```python
from build123d import *

# Parameters (mm, degrees)
SKETCH1_W           = 825.5
SKETCH1_H           = 825.5
SKETCH1_W_2         = 647.7
SKETCH1_H_2         = 647.7
BOSS_EXTRUDE1_DEPTH = 127
FILLET1_R           = 25.4
FILLET2_R           = 12.7
SKETCH2_W           = 34.200403136
SKETCH2_H           = 9.659395297
CUT_EXTRUDE1_DEPTH  = 5.08


with BuildPart() as part:
    # Sketch1 → Boss-Extrude1 (new body)
    with BuildSketch(Plane(origin=(0, 0, 0), x_dir=(1, 0, 0), z_dir=(0, 1, 0))):
        Rectangle(SKETCH1_W, SKETCH1_H)
        Rectangle(SKETCH1_W_2, SKETCH1_H_2, mode=Mode.SUBTRACT)
    extrude(amount=BOSS_EXTRUDE1_DEPTH)

    # Fillet1
    fillet1_edges = [part.edges().sort_by_distance(p)[0] for p in [
        (412.75, 63.5, 412.75),
        (-412.75, 63.5, 412.75),
        (-412.75, 63.5, -412.75),
        (412.75, 63.5, -412.75),
    ]]
    fillet(fillet1_edges, radius=FILLET1_R)

    # Fillet2
    fillet2_edges = [part.edges().sort_by_distance(p)[0] for p in [
        (-412.75, 0, 0),
        (-412.75, 127, 0),
        (412.75, 0, 0),
        (0, 0, 412.75),
        (0, 0, -412.75),
        (405.310512242, 0, 405.310512242),
        (405.310512242, 0, -405.310512242),
        (-405.310512242, 0, 405.310512242),
        (-405.310512242, 0, -405.310512242),
        (0, 127, -412.75),
        (412.75, 127, 0),
        (0, 127, 412.75),
        (405.310512242, 127, 405.310512242),
        (405.310512242, 127, -405.310512242),
        (-405.310512242, 127, 405.310512242),
        (-405.310512242, 127, -405.310512242),
    ]]
    fillet(fillet2_edges, radius=FILLET2_R)

    # Sketch2 → Cut-Extrude1 (cut)
    # profile 1 of 4: a face of its own
    with BuildSketch(Plane.ZY.offset(412.75)):
        Polygon((-121.32268757, 97.79), (-233.139574468, 97.79), (-211.090212766, 78.795464726), (-153.406898096, 78.795464726), (-153.406898096, 69.136069429), (-219.691511758, 69.136069429), (-219.691511758, 50.260996641), (-153.406898096, 50.260996641), (-153.406898096, 40.465072788), (-219.691511758, 40.465072788), (-219.691511758, 21.59), (-121.32268757, 21.59), align=None)
    # profile 2 of 4: a face of its own
    with BuildSketch(Plane.ZY.offset(412.75)):
        Polygon((-4.812631579, 97.79), (-116.271131019, 97.79), (-93.624456887, 78.795464726), (-48.928421053, 78.795464726), (-102.823068309, 21.59), (-59.065666293, 21.59), (-4.812631579, 78.795464726), align=None)
    # profile 3 of 4: a face of its own
    with BuildSketch(Plane.ZY.offset(412.75)):
        Polygon((80.329988802, 50.260996641), (80.329988802, 40.465072788), (14.147771557, 40.465072788), (14.147771557, 21.59), (112.294736842, 21.59), (112.294736842, 97.79), (0.59731243, 97.79), (14.147771557, 86.475195969), (14.147771557, 50.260996641), align=None)
        with Locations((63.229787234, 73.965767078)):
            Rectangle(SKETCH2_W, SKETCH2_H, mode=Mode.SUBTRACT)
    # profile 4 of 4: a face of its own
    with BuildSketch(Plane.ZY.offset(412.75)):
        Polygon((229.282642777, 97.79), (117.465755879, 97.79), (131.016215006, 86.475195969), (131.016215006, 78.795464726), (197.198432251, 78.795464726), (197.198432251, 69.136069429), (130.913818589, 69.136069429), (130.913818589, 21.59), (228.924255319, 21.59), (228.924255319, 40.465072788), (162.878566629, 40.465072788), (162.878566629, 50.260996641), (229.282642777, 50.260996641), align=None)
    extrude(amount=-CUT_EXTRUDE1_DEPTH, mode=Mode.SUBTRACT)


solid = part.part
```
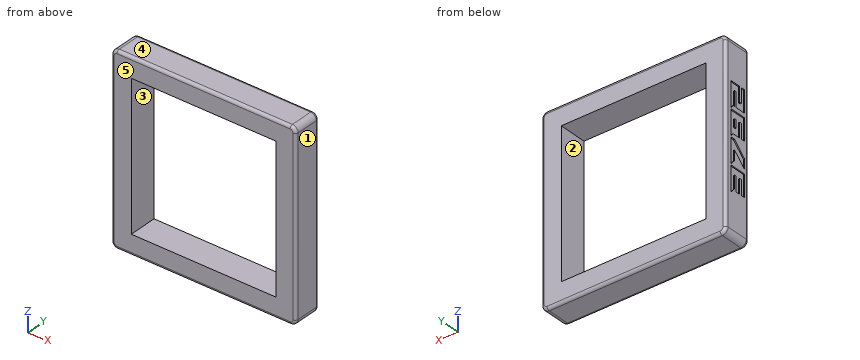
Geometry check sheet. Reference: the model listing, model coordinates, mm. Face numbers are marked on the shaded views. A direction names the side the tool comes from. Coordinates: 2 decimals unless noted, no trailing zeros. Write each loop counter-clockwise with the first axis right and the second up, starting at its lowest first coordinate (ties: lowest second). Pieces come first, ordered by that corner, then holes. Notation, with made-up numbers: M -21,26 L 5,26 A28 ccw 5,48 Z; hole C -10.75,-20 d5. An arc over 180 degrees is marked long. One line per item, written item: value. Start each with the question number.
(1) Depth check by flat-ended pin: pin 1 (1.5 mm diameter, centred on x = -410, z = 68, fed in from +Y) (3 decimals); pin 2 (4 mm diameter, centred on x = -409.5, y = 53, fed in from -Z); pin 3 (5.5 mm diameter, centred on x = -411, y = 64, fed in from +Z). Enter the tip coordinate at first touch or a pass-through.
(2) Release check for a two-part mould opening along Z. For the marked faces 3, 4 and 5 record: released by +Z, released by -Z, zero draft, split by the parting line, or undercut.
(3) Tool access check on the marked faces 1 and 2. Record the directions out of +Z, -Z, +X, -X, +Y, -Y that give a thin tool (end or side, any length) a straight path to the whole face; none if there is none.
(4) Sectioned sample at B-B, the plane z = -177. Enter the section's corners in (x, y), and give its area (3 significant figures).
(5) Sectioned sample at A-A, the plane x = 4.5. Enter the section's corners in (y, z), and give its area (3 significant figures).
(6) Scan lines: line 1 along Z through (x, y) = (-213, 12); line 2 along Z through (x, y) = (-203, 20). Record each from-to range of solid material in increasing order. Write a range as [from, to].
Filled sheet:
1. pin 1: y = 123.055
1. pin 2: z = -402.81
1. pin 3: z = 401.78
2. face 3: undercut
2. face 4: released by +Z
2. face 5: zero draft
3. face 1: +Z, -Z, +X, +Y, -Y
3. face 2: +Y, -Y
4. outline: M -412.75,12.7 A12.7 ccw -400.05,0 L -323.85,0 L -323.85,127 L -400.05,127 A12.7 ccw -412.75,114.3 L -412.75,97.79 L -407.67,97.79 L -407.67,78.8 L -412.75,78.8 L -412.75,69.14 L -407.67,69.14 L -407.67,50.26 L -412.75,50.26 L -412.75,40.47 L -407.67,40.47 L -407.67,21.59 L -412.75,21.59 Z; M 323.85,0 L 400.05,0 A12.7 ccw 412.75,12.7 L 412.75,114.3 A12.7 ccw 400.05,127 L 323.85,127 Z
4. area: 22,200 mm²
5. outline: M 0,-400.05 A12.7 ccw 12.7,-412.75 L 114.3,-412.75 A12.7 ccw 127,-400.05 L 127,-323.85 L 0,-323.85 Z; M 0,323.85 L 127,323.85 L 127,400.05 A12.7 ccw 114.3,412.75 L 12.7,412.75 A12.7 ccw 0,400.05 Z
5. area: 22,400 mm²
6. line 1: [-412.73, -323.85], [323.85, 412.73]
6. line 2: [-412.75, -323.85], [323.85, 412.75]
